The listing builds one solid part. Answer for the finished solid, in the listing's coordinates (mm). A direction names the side the tool comes from. Round coordinates to 2 decimals unless told otherwise and drop trailing zeros. Loops run counter-clockwise (first coordinate to the right, second up) from the corner with the lowest first, then second, coordinate; pieces in that order, holes last. Notation, with made-up numbers: (60, 28.5) -> (85, 28.5) arc R5 ccw to (85, 33.5) -> close; hole circle Ø11 at (14.25, -5). An arc over 180 degrees is marked (long way). Write each question's results on one line, items separated by ' | '. Start each with the question number.
from build123d import *

# Parameters (mm, degrees)
CROQUIS1_R              = 75
CROQUIS1_R_2            = 49
SALIENTE_EXTRUIR1_DEPTH = 5
CROQUIS2_R              = 1.7
CORTAR_EXTRUIR1_DEPTH   = 5
CROQUIS3_R              = 2.95
CORTAR_EXTRUIR2_DEPTH   = 3
MATRIZC1_COUNT          = 3


with BuildPart() as part:
    # Croquis1 → Saliente-Extruir1 (new body)
    with BuildSketch(Plane(origin=(0, 0, 0), x_dir=(1, 0, 0), z_dir=(0, 1, 0))):
        Circle(CROQUIS1_R)
        Circle(CROQUIS1_R_2, mode=Mode.SUBTRACT)
    extrude(amount=SALIENTE_EXTRUIR1_DEPTH)

    # Croquis2 → Cortar-Extruir1 (cut)
    with BuildSketch(Plane(origin=(0, 5, 0), x_dir=(1, 0, 0), z_dir=(0, 1, 0))):
        with Locations((-65, 0)):
            Circle(CROQUIS2_R)
    cortar_extruir1 = extrude(amount=-CORTAR_EXTRUIR1_DEPTH, mode=Mode.SUBTRACT)

    # Croquis3 → Cortar-Extruir2 (cut)
    with BuildSketch(Plane(origin=(0, 5, 0), x_dir=(1, 0, 0), z_dir=(0, 1, 0))):
        with Locations((-65, 0)):
            Circle(CROQUIS3_R)
    cortar_extruir2 = extrude(amount=-CORTAR_EXTRUIR2_DEPTH, mode=Mode.SUBTRACT)

    # MatrizC1: Cortar-Extruir1, Cortar-Extruir2 ×3 about axis
    matrizc1_axis = Axis((0, 0, 0), (0, 1, 0))
    for i in range(1, MATRIZC1_COUNT):
        add(cortar_extruir1.rotate(matrizc1_axis, i * 360 / MATRIZC1_COUNT), mode=Mode.SUBTRACT)
        add(cortar_extruir2.rotate(matrizc1_axis, i * 360 / MATRIZC1_COUNT), mode=Mode.SUBTRACT)


solid = part.part
Item 1: For faces 1 (the cylindrical face through (-66.7, 1.01, -0.07)), 2 (the flat face through (31.5, 2, 54.6)), determine the directions among +Z, -Z, +X, -X, +Y, -Y from which every point of the face is accessible in a straight line to the end or side of a thin tool.
Item 2: Straight lines are drawn through the part: L1, parallel to X at y = 3.9, z = 0; L2, parallel to Z at x = 32.5, y = 1.55; L3, parallel to Z at x = -0.5, y = 4.55. For each, find the intervals that lie inside material, in ascending order. Write a range as [from, to].
Item 3: The part is cut by section C-C, the plane z = 25. Give the vertices of the cut face in (x, y).
Item 4: Each of these flat-tipped pins is pushed along its axis until it touches: pin 1 Ø4.5 at (x, z) = (32.5, 56.29) entering from +Y; pin 2 Ø1.5 at (y, z) = (2, 18.5) entering from -X; pin 3 Ø3 at (x, z) = (-45.5, 1.5) entering from -Y. Where does it stop, or does it pass through?
Item 5: The part is cut by section D-D, the plane y = 4.25. Give the vertices of the cut face in (x, z) (3 decimals), plus the area to 3 significant figures.
Item 6: Determine the mould class of faces 3 (the flat face through (49, 0, 16)), 4 (the cylindrical face through (-9.764, 2.465, -74.362)), 5 (the cylindrical face through (32.131, 1.014, -54.632)) for opening direction X: +X half, -X half, draft (parallel to the pull), parting line (faces both ways), or undercut.
Item 7: The part is cut by section A-A, the plane x = 0. Give the vertices of the cut face in (y, z).
Item 8: The part is cut by section B-B, the plane z = 0. Give the vertices of the cut face in (x, y).
Report:
1) face 1: +Y, -Y | face 2: +Y
2) L1: x = [-75, -67.95], [-62.05, -49], [49, 75] | L2: z = [-67.59, -57.99], [-54.59, -36.67], [36.67, 54.59], [57.99, 67.59] | L3: z = [-75, -49], [49, 75]
3) outline: (-70.71, 0) -> (-42.14, 0) -> (-42.14, 5) -> (-70.71, 5) -> close; (42.14, 0) -> (70.71, 0) -> (70.71, 5) -> (42.14, 5) -> close
4) pin 1: stops at y = 2 | pin 2: stops at x = -72.87 | pin 3: passes through
5) outline: circle Ø150 at (0, 0); hole circle Ø5.9 at (-65, 0); hole circle Ø98 at (0, 0); hole circle Ø5.9 at (32.5, -56.292); hole circle Ø5.9 at (32.5, 56.292) | area: 10,000 mm2
6) face 3: draft | face 4: parting line | face 5: undercut
7) outline: (0, -75) -> (5, -75) -> (5, -49) -> (0, -49) -> close; (0, 49) -> (5, 49) -> (5, 75) -> (0, 75) -> close
8) outline: (-75, 0) -> (-66.7, 0) -> (-66.7, 2) -> (-67.95, 2) -> (-67.95, 5) -> (-75, 5) -> close; (-63.3, 0) -> (-49, 0) -> (-49, 5) -> (-62.05, 5) -> (-62.05, 2) -> (-63.3, 2) -> close; (49, 0) -> (75, 0) -> (75, 5) -> (49, 5) -> close
